from build123d import *

# Parameters (mm, degrees)
BOX_W       = 22
BOX_H       = 300
BOX_DEPTH   = 623
FILLET_R    = 18
FILLET001_R = 18


with BuildPart() as part:
    # Box → Box (new body)
    with BuildSketch(Plane.XY):
        with Locations((11, 150)):
            Rectangle(BOX_W, BOX_H)
    extrude(amount=BOX_DEPTH)

    # Fillet
    fillet_edges = [part.edges().sort_by_distance(p)[0] for p in [
        (0, 0, 311.5),
    ]]
    fillet(fillet_edges, radius=FILLET_R)

    # Fillet001
    fillet001_edges = [part.edges().sort_by_distance(p)[0] for p in [
        (0, 300, 311.5),
    ]]
    fillet(fillet001_edges, radius=FILLET001_R)


solid = part.part
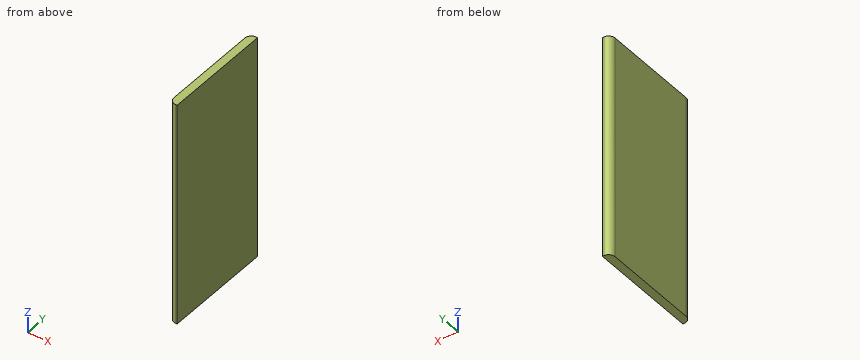
The listing builds one solid part. Answer for the finished solid, in the listing's coordinates (mm). Round coordinates to 2 decimals unless told otherwise and drop trailing zeros. Order: outer loops, then holes, each group sorted by start corner. A loop starts at its lowest first (then second) coordinate and runs counter-clockwise, first axis right, second up. Notation, with made-up numbers: M 24,5 L 80,5 A18 cw 80,37 Z; hole C 25,72.5 d1. An arc over 180 degrees is marked long. Answer in a Markdown table with one row per item. Add a question column.
1) Consider line 1 along Y through (x, z) = (17.75, 98.5); line 2 along Y through (x, z) = (4.5, 84). Determine where each line is inside the solid, lowest interval first. Write a range as from..to.
2) Flat-ended cylindrical pins translate along their axes: pin 1 Ø3 at (x, z) = (17.5, 252) entering from +Y; pin 2 Ø1 at (x, z) = (4.5, 539.5) entering from +Y; pin 3 Ø1.5 at (x, z) = (10.5, 320) entering from +Y. Find the tip coordinate at first contact, or state that the pin passes through.
3) The part is cut by section B-B on x = 8. Determine the outline of the cut face in (y, z), plus the area to 3 significant figures.
4) The part is cut by section A-A on z = 569.5. Determine the outline of the cut face in (x, y).
Findings below:
| question | item | result |
|---|---|---|
| 1 | line 1 | y = 0..300 |
| 1 | line 2 | y = 6.09..293.91 |
| 2 | pin 1 | stops at y = 300 |
| 2 | pin 2 | stops at y = 294.45 |
| 2 | pin 3 | stops at y = 298.69 |
| 3 | outline | M 3.03,0 L 296.97,0 L 296.97,623 L 3.03,623 Z |
| 3 | area | 183,000 mm² |
| 4 | outline | M 0,18 A18 ccw 18,0 L 22,0 L 22,300 L 18,300 A18 ccw 0,282 Z |
